Design review of the part built by this model. Coordinates are the model's own, in mm. A direction names the side the tool comes from. Round coordinates to 2 decimals unless told otherwise and drop trailing zeros. Loops run counter-clockwise (first coordinate to the right, second up) from the corner with the lowest first, then second, coordinate; pieces in that order, holes last. Notation, with made-up numbers: M 21,7 L 33,7 A22 cw 33,22 Z; hole C -13.5,88 d6. An arc over 180 degrees is marked long. Answer as CSV lines item,"result". Start each with the question number.
from build123d import *

# Parameters (mm, degrees)
F0_W     = 63.5
F0_H     = 63.5
F1_DEPTH = 63.5
F2_W     = 50.8
F2_H     = 50.8
F3_DEPTH = 50.893329
F4_W     = 12.7
F4_H     = 12.7
F5_DEPTH = 25.4


with BuildPart() as f1:
    # F0 (on Front) → F1 (new body)
    with BuildSketch(Plane.XZ):
        with Locations((31.75, 31.75)):
            Rectangle(F0_W, F0_H)
    extrude(amount=F1_DEPTH)

    # F2 (on face) → F3 (cut)
    with BuildSketch(Plane.XY.offset(63.5)):
        with Locations((38.1, -38.1)):
            Rectangle(F2_W, F2_H)
    extrude(amount=-F3_DEPTH, mode=Mode.SUBTRACT)

    # F4 (on face) → F5 (cut)
    with BuildSketch(Plane.XY.offset(12.606671)):
        with Locations((57.15, -57.15)):
            Rectangle(F4_W, F4_H)
    extrude(amount=-F5_DEPTH, mode=Mode.SUBTRACT)


solid = f1.part
Item 1: Consider section B-B, the plane y = -29.5. Write out the cut boundary in (x, z).
Item 2: To check wall thickness, follow line 1 (Y direction, x = 25.5, z = 22); line 2 (Z direction, x = 46.5, y = -15.5); line 3 (X direction, y = -31, z = 45.5). State the ranges of each line that lie inside material, in increasing order.
Item 3: Tool access review of faces 1 (the face through (38, -12.7, 38)), 2 (the face through (31, 0, 32)), 3 (the face through (50.8, -57, 6)): name each direction out of +Z, -Z, +X, -X, +Y, -Y from which nothing blocks a thin tool from reaching the whole face with its end or side.
Item 4: Insertion check: pin 1 Ø6 at (x, z) = (54, 43) entering from +Y; pin 2 Ø8 at (x, y) = (50, -56) entering from +Z; pin 3 Ø4 at (y, z) = (-16, 35) entering from +X; pin 4 Ø15 at (x, z) = (30.5, 46.5) entering from -Y. Each pin has a flat end and moves straight along its axis. Give the tip position at first contact, or say it passes through.
Item 5: Consider section A-A, the plane z = 16.5. Write out the cut boundary in (x, y).
Found:
1,outline,"M 0,0 L 63.5,0 L 63.5,12.61 L 12.7,12.61 L 12.7,63.5 L 0,63.5 Z"
2,line 1,"y = -12.7 to 0"
2,line 2,"z = 0 to 12.61"
2,line 3,"x = 0 to 12.7"
3,face 1,"+Z, +X, -Y"
3,face 2,"+Z, -Z, +X, -X, +Y"
3,face 3,"+Z, -Z, +X, -Y"
4,pin 1,"stops at y = 0"
4,pin 2,"stops at z = 12.61"
4,pin 3,"stops at x = 12.7"
4,pin 4,"stops at y = -12.7"
5,outline,"M 0,-63.5 L 12.7,-63.5 L 12.7,-12.7 L 63.5,-12.7 L 63.5,0 L 0,0 Z"
